Design review of the part built by this model. Coordinates are the model's own, in mm. Coordinates: 2 decimals unless noted, no trailing zeros. Write each loop counter-clockwise with the first axis right and the second up, starting at its lowest first coordinate (ties: lowest second). Pieces come first, ordered by that corner, then holes.
Q1. Add section C-C, the plane x = 30. Give the boundary of the cut face in (y, z), plus the area to 3 significant figures.
Q2. Add section D-D, the plane z = 1.65. Give the boundary of the cut face in (x, y), plus the area to 3 significant figures.
Q3. Add section B-B, the plane x = 10. Give the boundary of the cut face in (y, z).
Q4. To check wall thickness, follow probe 1 along Y at (x, z) = (10, 0.65); probe 2 along Y at (x, z) = (-0.5, 1.25); probe 3 along X at (y, z) = (34, 1.35). State the ranges of each line that lie inside material, in increasing order.
Q5. Add section A-A, the plane y = 20. Give the boundary of the cut face in (x, z).
Q6. Clearance check with a flat-ended pin moving along its axis: pin 1 Ø1 at (y, z) = (27, 2) entering from +X (3 decimals). State where the tip first meets the part, or that it passes through.
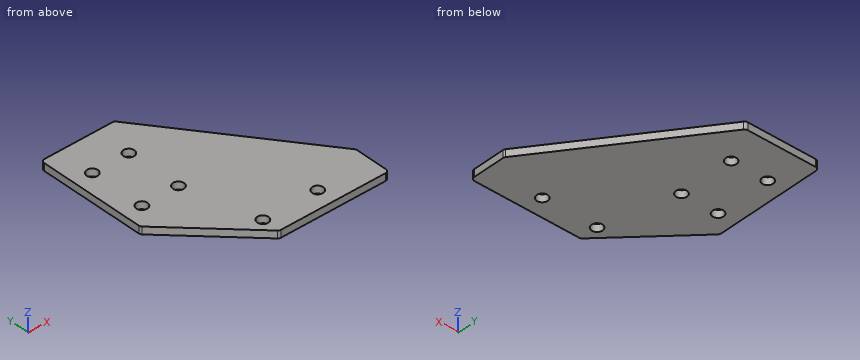
from build123d import *

# Parameters (mm, degrees)
SKETCH_1_R      = 1.5
EXTRUDE_1_DEPTH = 2
FILLET_1_R      = 1


with BuildPart() as part:
    # 草图1 → 凸台-拉伸1 (new body)
    with BuildSketch(Plane.XY):
        Polygon((-5, 45), (15, 45), (45, 5), (45, -5), (15, -5), (-5, 15), align=None)
        with Locations((0, 35)):
            Circle(SKETCH_1_R, mode=Mode.SUBTRACT)
        with Locations((30, 0)):
            Circle(SKETCH_1_R, mode=Mode.SUBTRACT)
        with Locations((0, 20)):
            Circle(SKETCH_1_R, mode=Mode.SUBTRACT)
        with Locations((15, 0)):
            Circle(SKETCH_1_R, mode=Mode.SUBTRACT)
        with Locations((10, 35)):
            Circle(SKETCH_1_R, mode=Mode.SUBTRACT)
        with Locations((10, 20)):
            Circle(SKETCH_1_R, mode=Mode.SUBTRACT)
    extrude(amount=EXTRUDE_1_DEPTH)

    # 圆角1
    fillet_1_edges = [part.edges().sort_by_distance(p)[0] for p in [
        (-5, 45, 1),
        (15, 45, 1),
        (45, 5, 1),
        (45, -5, 1),
        (15, -5, 1),
        (-5, 15, 1),
    ]]
    fillet(fillet_1_edges, radius=FILLET_1_R)


solid = part.part
Here are the results:
1. outline: (-5, 0) - (-1.5, 0) - (-1.5, 2) - (-5, 2) - close; (1.5, 0) - (25, 0) - (25, 2) - (1.5, 2) - close
1. area: 54.0 mm2
2. outline: (-5, 15.41) arc R1 ccw to (-4.71, 14.71) - (14.71, -4.71) arc R1 ccw to (15.41, -5) - (44, -5) arc R1 ccw to (45, -4) - (45, 4.67) arc R1 ccw to (44.8, 5.27) - (15.3, 44.6) arc R1 ccw to (14.5, 45) - (-4, 45) arc R1 ccw to (-5, 44) - close; hole circle Ø3 at (0, 20); hole circle Ø3 at (0, 35); hole circle Ø3 at (10, 20); hole circle Ø3 at (10, 35); hole circle Ø3 at (15, 0); hole circle Ø3 at (30, 0)
2. area: 1,660 mm2
3. outline: (0, 0) - (18.5, 0) - (18.5, 2) - (0, 2) - close; (21.5, 0) - (33.5, 0) - (33.5, 2) - (21.5, 2) - close; (36.5, 0) - (45, 0) - (45, 2) - (36.5, 2) - close
4. probe 1: y = 0 to 18.5, 21.5 to 33.5, 36.5 to 45
4. probe 2: y = 10.5 to 18.59, 21.41 to 33.59, 36.41 to 45
4. probe 3: x = -5 to -1.12, 1.12 to 8.88, 11.12 to 23.25
5. outline: (-5, 0) - (-1.5, 0) - (-1.5, 2) - (-5, 2) - close; (1.5, 0) - (8.5, 0) - (8.5, 2) - (1.5, 2) - close; (11.5, 0) - (33.75, 0) - (33.75, 2) - (11.5, 2) - close
6. pin 1: stops at x = 28.875
